Design review of the part built by this model. Coordinates are the model's own, in mm. A direction names the side the tool comes from. Round coordinates to 2 decimals unless told otherwise and drop trailing zeros. Write each loop counter-clockwise with the first axis right and the second up, starting at its lowest first coordinate (ties: lowest second). Pieces come first, ordered by that corner, then holes. Notation, with made-up numbers: M 26.5,2.5 L 41.5,2.5 A32 cw 41.5,38.5 Z; hole C 57,61 d9. An arc over 180 degrees is marked long. One line per question, with ' | ' between items. Start each with the question number.
Item 1: Add section A-A, the plane y = 0. State the section outline as (x, z) points (3 decimals), and give its area (3 significant figures).
Item 2: Add section C-C, the plane y = 12.7. Give the number of separate pieces and of enclosed holes in the cut face, and give its area (3 significant figures).
Item 3: Draft analysis for pull direction Y (two halves, no side actions). For faces 3 (the face through (14.5, -14.5, 12.7)), 4 (the face through (4.13, 18.597, 22.109)), 5 (the face through (18.825, 12.56, 6.261)), state which applies: released by +Y, released by -Y, zero draft, split by the parting line, or undercut.
Item 4: For L1, parallel to Y at x = 0, z = 15 (3 decimals); L2, parallel to Y at x = 0, z = 12 (3 decimals); L3, parallel to X at y = 12, z = 4, list the stretches that pass through material, from the lowest coordinate up.
Item 5: Machinability: for faces 1 (the face through (8.454, 12.935, 23.564)), 2 (the face through (3.23, 10.36, 15.65)), which of the approach directions +Z, -Z, +X, -X, +Y, -Y give a long, thin tool a straight path to every point of the face, cutting with its end or side? Answer none if there is none.
Item 6: Insertion check: pin 1 Ø12 at (x, y) = (18.5, 17) entering from +Z; pin 2 Ø4 at (y, z) = (3.5, 11.5) entering from +X; pin 3 Ø1.5 at (x, z) = (20, 18) entering from -Y; pin 4 Ø8.5 at (x, y) = (0, 25.4) entering from +Z. Each pin has a flat end and moves straight along its axis. Give the tip position at first contact, or say it passes through.
```python
from build123d import *

# Parameters (mm, degrees)
SKETCH1_R          = 34.925
EXTRUDE1_DEPTH     = 12.7
SKETCH2_R          = 19.05
EXTRUDE2_DEPTH     = 19.05
SKETCH3_R          = 3.175
SKETCH3_R_2        = 9.525
CUT_EXTRUDE1_DEPTH = 59.716043378
CIRPATTERN1_COUNT  = 6
CUT_EXTRUDE2_DEPTH = 59.716043378
SKETCH5_R          = 1.5875
CUT_EXTRUDE3_DEPTH = 69.74147002
CHAMFER1_SIZE      = 1.27


with BuildPart() as part:
    # Sketch1 → Extrude1 (new body)
    with BuildSketch(Plane.XY):
        Circle(SKETCH1_R)
    extrude(amount=EXTRUDE1_DEPTH)

    # Sketch2 → Extrude2 (add)
    with BuildSketch(Plane.XY.offset(12.7)):
        with Locations(Location((0, 0, 0), (0, 0, 180))):
            Circle(SKETCH2_R)
    extrude(amount=EXTRUDE2_DEPTH)

    # Sketch3 → Cut-Extrude1 (cut, through all)
    with BuildSketch(Plane(origin=(0, 0, 0), x_dir=(-1, 0, 0), z_dir=(0, 0, -1))):
        with Locations((0, 25.4)):
            Circle(SKETCH3_R)
        Circle(SKETCH3_R_2)
    cut_extrude1 = extrude(amount=-CUT_EXTRUDE1_DEPTH, mode=Mode.SUBTRACT)

    # CirPattern1: Cut-Extrude1 ×6 about axis
    cirpattern1_axis = Axis((0, 0, 0), (0, 0, 1))
    for i in range(1, CIRPATTERN1_COUNT):
        add(cut_extrude1.rotate(cirpattern1_axis, i * 360 / CIRPATTERN1_COUNT), mode=Mode.SUBTRACT)

    # Sketch4 → Cut-Extrude2 (cut, through all)
    with BuildSketch(Plane(origin=(0, 0, 0), x_dir=(-1, 0, 0), z_dir=(0, 0, -1))):
        Polygon((-1.509652007, 7.377293978), (-5.634097993, 4.996043978), (-8.015347993, 9.120489964), (-3.890902007, 11.501739964), align=None)
    extrude(amount=-CUT_EXTRUDE2_DEPTH, mode=Mode.SUBTRACT)

    # Sketch5 → Cut-Extrude3 (cut, through all)
    with BuildSketch(Plane(origin=(5.953125, 10.311114964, 0), x_dir=(0.8660254037844396, -0.4999999999999984, 0), z_dir=(-0.4999999999999984, -0.8660254037844396, 0))):
        with Locations((0, 22.225)):
            Circle(SKETCH5_R)
    extrude(amount=-CUT_EXTRUDE3_DEPTH, mode=Mode.SUBTRACT)

    # Chamfer1
    chamfer1_edges = [part.edges().sort_by_distance(p)[0] for p in [
        (-34.925, 0, 12.7),
        (19.05, 0, 12.7),
        (19.05, 0, 31.75),
    ]]
    chamfer(chamfer1_edges, length=CHAMFER1_SIZE)


solid = part.part
```
Computed values:
1) outline: M -34.925,0 L -9.525,0 L -9.525,31.75 L -17.78,31.75 L -19.05,30.48 L -19.05,13.97 L -20.32,12.7 L -33.655,12.7 L -34.925,11.43 Z; M 9.525,0 L 34.925,0 L 34.925,11.43 L 33.655,12.7 L 20.32,12.7 L 19.05,13.97 L 19.05,30.48 L 17.78,31.75 L 9.525,31.75 Z | area: 1,010 mm^2
2) separate pieces: 3 | enclosed holes: 1 | area: 1,200 mm^2
3) face 3: zero draft | face 4: split by the parting line | face 5: undercut
4) L1: y = -19.05 to -9.525, 9.525 to 19.05 | L2: y = -34.355 to -28.575, -22.225 to -9.525, 9.525 to 22.225, 28.575 to 34.355 | L3: x = -32.8 to -25.09, -18.9 to 18.9, 25.09 to 32.8
5) face 1: none | face 2: +Z, -Z
6) pin 1: stops at z = 13.9 | pin 2: stops at x = 34.89 | pin 3: passes through | pin 4: stops at z = 12.7
